Study the drawing (mm; zero at the part's minimum x, y, z) and answer. Coordinates: 2 decimals unless noted, no trailing zeros. Loops run counter-clockwise (first coordinate to the right, second up) from the corner with the lowest first, then second, coordinate; pieces in that order, holes last. Notation, with made-up numbers: (-3.5, -32) -> (37.5, -32) arc R20 ccw to (37.5, -24) -> close; hole circle Ø7 at (53.5, -11.75). An arc over 180 degrees is marked (long way). Answer in a Markdown table with one row per item.
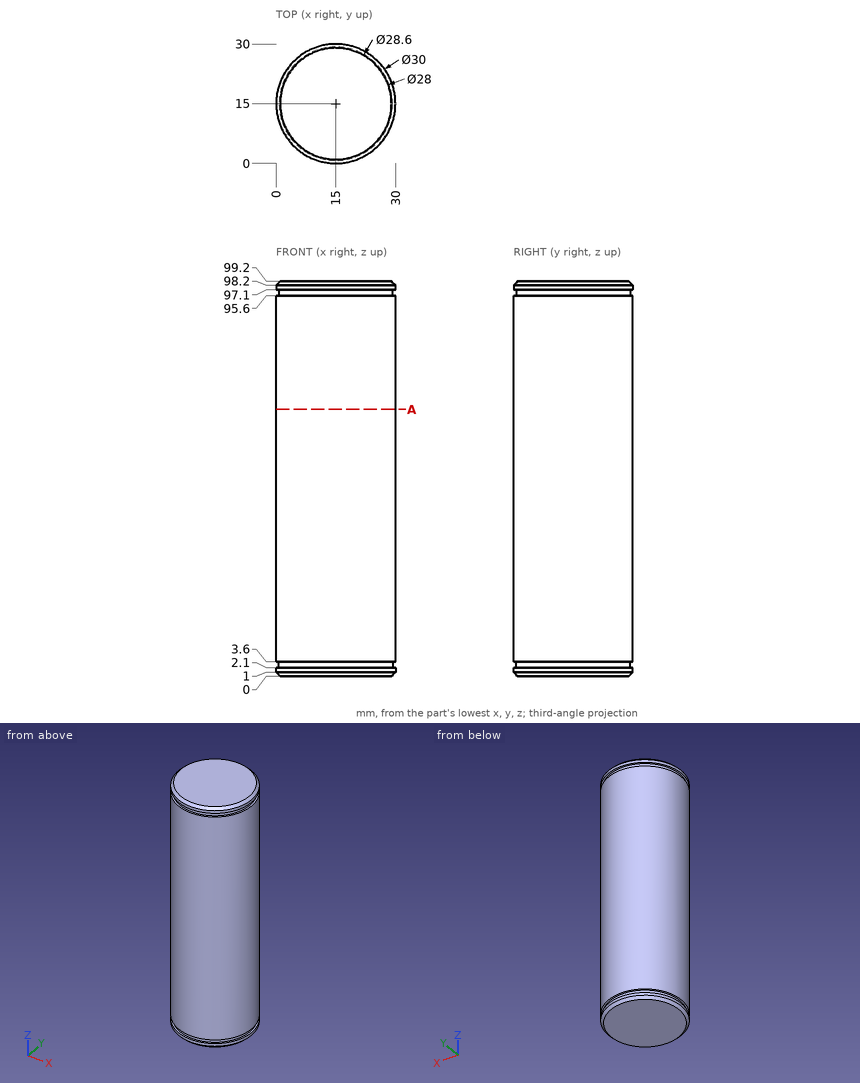
1. A cutting plane is placed at A-A on z = 67. Give the vertices of the cut face in (x, y).
A:
| item | result |
|---|---|
| outline | circle Ø30 at (15, 15) |
2. Given pin 1 Ø5 at (x, z) = (4, 78) entering from -Y; pin 2 Ø1.5 at (x, z) = (9, 80) entering from +Y; pin 3 Ø3 at (y, z) = (7.5, 63) entering from +X, each flat-ended and moving along its own axis, determine where each tip first touches the part or whether it passes through.
A:
| item | result |
|---|---|
| pin 1 | stops at y = 2.64 |
| pin 2 | stops at y = 29.05 |
| pin 3 | stops at x = 28.75 |
3. Find the intervals of material crossed by probe 1 along Z at (x, y) = (27.75, 21.75); probe 2 along Y at (x, z) = (15, 72.5); probe 3 along Z at (x, y) = (15.75, 29), in increasing order.
A:
| item | result |
|---|---|
| probe 1 | z = 0.43 to 2.1, 3.6 to 95.6, 97.1 to 98.77 |
| probe 2 | y = 0 to 30 |
| probe 3 | z = 0.02 to 99.18 |
